Geometry check sheet. Reference: the model listing, model coordinates, mm. A direction names the side the tool comes from. Give positions to 0.01 mm unless a question says otherwise; leave off trailing zeros. Loops run counter-clockwise (first coordinate to the right, second up) from the corner with the lowest first, then second, coordinate; pieces in that order, holes last. Notation, with made-up numbers: (-39.5, 52.5) - (11.5, 52.5) arc R37 ccw to (11.5, 88.5) - close; hole circle Ø6 at (54, 83.25). An arc over 180 degrees is marked (long way). Use a Markdown table: item, result. Add a question column.
1. Cross-section at D-D on x = -22.5. Enter the section's corners in (y, z), and give its area (3 significant figures).
2. Depth check by flat-ended pin: P1, Ø8, axis at y = 23.5, z = 2, coming from the +X side; P2, Ø3, axis at y = 14, z = -11, coming from the -X side; P3, Ø3.5, axis at x = 28.5, y = 10, coming from the -Z side. Enter the tip coordinate at first touch or a pass-through.
3. Cross-section at A-A on z = 0. Enter the section's corners in (x, y), and give its area (3 significant figures).
4. Cross-section at C-C on x = 0. Enter the section's corners in (y, z).
5. Material ranges on L1, parallel to X at y = 8.5, z = 0; L2, parallel to Z at x = -24, y = 3.5; L3, parallel to X at y = 9, z = 10.5, recorded low to high.
6. Set-up check for faces 1 (the flat face through (21, 18, 0)), 2 (the flat face through (-27, 17, 16)), 3 (the flat face through (0, 17, -21)): record each of +Z, -Z, +X, -X, +Y, -Y from which the full face is reachable in a straight line by a thin tool's end or side.
7. Cross-section at B-B on y = 27.5. Enter the section's corners in (x, z), and give its area (3 significant figures).
from build123d import *

# Parameters (mm, degrees)
SKETCH3_W           = 55
SKETCH3_H           = 42
BOSS_EXTRUDE1_DEPTH = 35
SKETCH4_R           = 16
CUT_EXTRUDE1_DEPTH  = 35
SKETCH5_W           = 6.5
SKETCH5_H           = 37
CUT_EXTRUDE2_DEPTH  = 35
FILLET1_R           = 5
SKETCH6_W           = 5
SKETCH6_H           = 35
BOSS_EXTRUDE2_DEPTH = 5
SKETCH7_W           = 5
SKETCH7_H           = 35
BOSS_EXTRUDE3_DEPTH = 5


with BuildPart() as part:
    # Sketch3 → Boss-Extrude1 (new body)
    with BuildSketch(Plane(origin=(0, 0, 0), x_dir=(1, 0, 0), z_dir=(0, 1, 0))):
        Rectangle(SKETCH3_W, SKETCH3_H)
    extrude(amount=BOSS_EXTRUDE1_DEPTH)

    # Sketch4 → Cut-Extrude1 (cut)
    with BuildSketch(Plane(origin=(0, 35, 0), x_dir=(1, 0, 0), z_dir=(0, 1, 0))):
        with Locations(Location((0, 0, 0), (0, 0, 270))):
            Circle(SKETCH4_R)
    extrude(amount=-CUT_EXTRUDE1_DEPTH, mode=Mode.SUBTRACT)

    # Sketch5 → Cut-Extrude2 (cut)
    with BuildSketch(Plane(origin=(0, 35, 0), x_dir=(1, 0, 0), z_dir=(0, 1, 0))):
        with Locations((-24.25, 2.5)):
            Rectangle(SKETCH5_W, SKETCH5_H)
        with Locations((24.25, 2.5)):
            Rectangle(SKETCH5_W, SKETCH5_H)
    extrude(amount=-CUT_EXTRUDE2_DEPTH, mode=Mode.SUBTRACT)

    # Fillet1
    fillet1_edges = [part.edges().sort_by_distance(p)[0] for p in [
        (-21, 17.5, -21),
        (21, 17.5, -21),
    ]]
    fillet(fillet1_edges, radius=FILLET1_R)

    # Sketch6 → Boss-Extrude2 (add)
    with BuildSketch(Plane(origin=(27.5, 0, 0), x_dir=(0, 0, -1), z_dir=(1, 0, 0))):
        with Locations((-18.5, 17.5)):
            Rectangle(SKETCH6_W, SKETCH6_H)
    extrude(amount=BOSS_EXTRUDE2_DEPTH)

    # Sketch7 → Boss-Extrude3 (add)
    with BuildSketch(Plane.ZY.offset(27.5)):
        with Locations((18.5, 17.5)):
            Rectangle(SKETCH7_W, SKETCH7_H)
    extrude(amount=BOSS_EXTRUDE3_DEPTH)


solid = part.part
Values found:
| question | item | result |
|---|---|---|
| 1 | outline | (0, 16) - (35, 16) - (35, 21) - (0, 21) - close |
| 1 | area | 175 mm2 |
| 2 | P1 | stops at x = 21 |
| 2 | P2 | stops at x = -21 |
| 2 | P3 | stops at z = 16 |
| 3 | outline | (-21, 0) - (-16, 0) - (-16, 35) - (-21, 35) - close; (16, 0) - (21, 0) - (21, 35) - (16, 35) - close |
| 3 | area | 350 mm2 |
| 4 | outline | (0, -21) - (35, -21) - (35, -16) - (0, -16) - close; (0, 16) - (35, 16) - (35, 21) - (0, 21) - close |
| 5 | L1 | x = -21 to -16, 16 to 21 |
| 5 | L2 | z = 16 to 21 |
| 5 | L3 | x = -21 to -12.07, 12.07 to 21 |
| 6 | face 1 | -Z, +X, +Y, -Y |
| 6 | face 2 | -Z, -X, +Y, -Y |
| 6 | face 3 | -Z, +X, -X, +Y, -Y |
| 7 | outline | (-32.5, 16) - (-21, 16) - (-21, -16) arc R5 ccw to (-16, -21) - (16, -21) arc R5 ccw to (21, -16) - (21, 16) - (32.5, 16) - (32.5, 21) - (-32.5, 21) - close; hole circle Ø32 at (0, 0) |
| 7 | area | 1,060 mm2 |
